Verification items for the finished model (mm, model axes). A direction names the side the tool comes from. Give positions to 0.01 mm unless a question says otherwise; leave off trailing zeros. Order: outer loops, then holes, each group sorted by start corner. A loop starts at its lowest first (then second) coordinate and runs counter-clockwise, first axis right, second up. Notation, with made-up numbers: (22, 83.25) -> (66, 83.25) arc R21 ccw to (66, 88.25) -> close; hole circle Ø4 at (70, -40). An arc over 180 degrees is marked (long way). One line per question, with ' | ' between items. Start each with the question number.
Q1. Section check C-C on z = 12.5. Record the cut outline in (x, y).
Q2. Mould release check, pull along Y, two halves, no side actions. Record for faces 1 (the flat face through (4.623, 7.515, 7.395)), 2 (the flat face through (-8.3, -3, 7)), 3 (the cylindrical face through (-6.77, 10.01, 7.4)): released by +Y, released by -Y, zero draft, split by the parting line, or undercut.
Q3. Access from +Z, -Z, +X, -X, +Y, -Y to the whole of each face (thin tool, end or side, straight path). Record for faces 4 (the flat face through (-1.3, -7, 7)), 5 (the flat face through (-2, -3.1, 7)), 6 (the flat face through (12.263, 9.56, 7.395)).
Q4. Section check D-D on x = -4. Record the cut outline in (y, z).
Q5. Section check B-B on y = 8.5. Record the cut outline in (x, z).
Q6. Section check A-A on y = -4.75. Record the cut outline in (x, z), plus the area to 3 significant figures.
Q7. Material ranges on probe 1 along X at (y, z) = (1, 2.25); probe 2 along X at (y, z) = (-7.5, 8.75); probe 3 along Y at (x, z) = (-6.5, 6.75), recorded low to high. Write a range as [from, to].
Q8. Go/stop test with flat-tipped pins: pin 1 (1.6 mm diameter, centred on x = -2.5, z = 6, fed in from +Y); pin 2 (1.2 mm diameter, centred on y = 2, z = 10.5, fed in from +X); pin 3 (7.5 mm diameter, centred on y = -7.5, z = 8, fed in from +X). Record where each tip stops, or that it passes through.
from build123d import *

# Parameters (mm, degrees)
F0_W     = 2
F0_H     = 4
F1_DEPTH = 15
F2_W     = 2
F2_H     = 4
F3_DEPTH = 15


# Not quite as in the source:
# - a feature names something its author has since deleted; it is built from what else it names


with BuildPart() as f1:
    # F0 (on Top) → F1 (new body)
    with BuildSketch(Plane.XY):
        with BuildLine():
            Line((7, 32.0000030547), (2, 32.0000030547))
            Line((2, 32.0000030547), (2, 43.0000030547))
            ThreePointArc((2, 43.0000030547), (4.22965477, 48.1459058579), (9.7375987459, 49.20147642))
            Line((9.7375987459, 49.20147642), (10.3227891625, 51.113949211))
            ThreePointArc((10.3227891625, 51.113949211), (3.4424209582, 50.0513163902), (0, 44.0000030547))
            Line((0, 44.0000030547), (0, 30.0000030547))
            Line((0, 30.0000030547), (9, 30.0000030547))
            Line((9, 30.0000030547), (9, 37.0000030547))
            Line((9, 37.0000030547), (7, 37.0000030547))
            Line((7, 37.0000030547), (7, 32.0000030547))
        make_face()
        Polygon((10.3227891625, 51.113949211), (9.7375987459, 49.20147642), (20.2561990964, 45.9829291287), (20.841389513, 47.8954019197), align=None)
        with BuildLine():
            Line((20.841389513, 47.8954019197), (20.2561990964, 45.9829291287))
            ThreePointArc((20.2561990964, 45.9829291287), (20.7938383415, 45.6028219427), (21, 44.9774941877))
            Line((21, 44.9774941877), (23, 44.9774941877))
            ThreePointArc((23, 44.9774941877), (22.9273260191, 45.6394915882), (22.7127657141, 46.2699564496))
            ThreePointArc((22.7127657141, 46.2699564496), (22.1205825647, 47.1207678466), (21.277739528, 47.7242382529))
            ThreePointArc((21.277739528, 47.7242382529), (21.0628558439, 47.8182107047), (20.841389513, 47.8954019197))
        make_face()
        with Locations((22, 42.9774941877)):
            Rectangle(F0_W, F0_H)
        with BuildLine():
            Line((23.8132360697, 51.5414804224), (21.277739528, 47.7242382529))
            ThreePointArc((21.277739528, 47.7242382529), (22.1205825647, 47.1207678466), (22.7127657141, 46.2699564496))
            Line((22.7127657141, 46.2699564496), (25.4792139424, 50.4349011311))
            Line((25.4792139424, 50.4349011311), (23.8132360697, 51.5414804224))
        make_face()
    extrude(amount=F1_DEPTH)


with BuildPart() as f3:
    # F2 (on Top) → F3 (new body)
    with BuildSketch(Plane.XY):
        with Locations((-37.8, -36.9225088671)):
            Rectangle(F2_W, F2_H)
        with BuildLine():
            ThreePointArc((-39.5438009036, -33.9170739261), (-39.0061616585, -34.2971811121), (-38.8, -34.9225088671))
            Line((-38.8, -34.9225088671), (-36.8, -34.9225088671))
            ThreePointArc((-36.8, -34.9225088671), (-36.8726739809, -34.2605114665), (-37.0872342859, -33.6300466052))
            ThreePointArc((-37.0872342859, -33.6300466052), (-37.6794174353, -32.7792352081), (-38.522260472, -32.1757648018))
            ThreePointArc((-38.522260472, -32.1757648018), (-38.7371441561, -32.0817923501), (-38.958610487, -32.0046011351))
            Line((-38.958610487, -32.0046011351), (-39.5438009036, -33.9170739261))
        make_face()
        Polygon((-50.0624012541, -30.6985266348), (-39.5438009036, -33.9170739261), (-38.958610487, -32.0046011351), (-49.4772108375, -28.7860538438), align=None)
        with BuildLine():
            ThreePointArc((-57.8, -36.9), (-55.57034523, -31.7540971969), (-50.0624012541, -30.6985266348))
            Line((-50.0624012541, -30.6985266348), (-49.4772108375, -28.7860538438))
            ThreePointArc((-49.4772108375, -28.7860538438), (-56.3575790418, -29.8486866645), (-59.8, -35.9))
            Line((-59.8, -35.9), (-59.8, -49.9))
            Line((-59.8, -49.9), (-50.8, -49.9))
            Line((-50.8, -49.9), (-50.8, -42.9))
            Line((-50.8, -42.9), (-52.8, -42.9))
            Line((-52.8, -42.9), (-52.8, -47.9))
            Line((-52.8, -47.9), (-57.8, -47.9))
            Line((-57.8, -47.9), (-57.8, -36.9))
        make_face()
        with BuildLine():
            ThreePointArc((-38.522260472, -32.1757648018), (-37.6794174353, -32.7792352081), (-37.0872342859, -33.6300466052))
            Line((-37.0872342859, -33.6300466052), (-34.3207860576, -29.4651019236))
            Line((-34.3207860576, -29.4651019236), (-35.9867639303, -28.3585226323))
            Line((-35.9867639303, -28.3585226323), (-38.522260472, -32.1757648018))
        make_face()
    extrude(amount=F3_DEPTH)


with BuildPart() as f3b:
    # F2 (on Top) → F3, piece 2 (new body)
    with BuildSketch(Plane.XY):
        with Locations((33.034186706, 0.0025241677)):
            Rectangle(F2_W, F2_H)
        with BuildLine():
            ThreePointArc((31.2903858024, 3.0079591087), (31.8280250475, 2.6278519227), (32.034186706, 2.0025241677))
            Line((32.034186706, 2.0025241677), (34.034186706, 2.0025241677))
            ThreePointArc((34.034186706, 2.0025241677), (33.9615127251, 2.6645215683), (33.7469524201, 3.2949864296))
            ThreePointArc((33.7469524201, 3.2949864296), (33.1547692707, 4.1457978267), (32.311926234, 4.749268233))
            ThreePointArc((32.311926234, 4.749268233), (32.0970425499, 4.8432406847), (31.875576219, 4.9204318997))
            Line((31.875576219, 4.9204318997), (31.2903858024, 3.0079591087))
        make_face()
        Polygon((20.7717854519, 6.2265064), (31.2903858024, 3.0079591087), (31.875576219, 4.9204318997), (21.3569758685, 8.138979191), align=None)
        with BuildLine():
            ThreePointArc((13.034186706, 0.0250330348), (15.2638414761, 5.1709358379), (20.7717854519, 6.2265064))
            Line((20.7717854519, 6.2265064), (21.3569758685, 8.138979191))
            ThreePointArc((21.3569758685, 8.138979191), (14.4766076642, 7.0763463703), (11.034186706, 1.0250330348))
            Line((11.034186706, 1.0250330348), (11.034186706, -12.9749669652))
            Line((11.034186706, -12.9749669652), (20.034186706, -12.9749669652))
            Line((20.034186706, -12.9749669652), (20.034186706, -5.9749669652))
            Line((20.034186706, -5.9749669652), (18.034186706, -5.9749669652))
            Line((18.034186706, -5.9749669652), (18.034186706, -10.9749669652))
            Line((18.034186706, -10.9749669652), (13.034186706, -10.9749669652))
            Line((13.034186706, -10.9749669652), (13.034186706, 0.0250330348))
        make_face()
        with BuildLine():
            ThreePointArc((32.311926234, 4.749268233), (33.1547692707, 4.1457978267), (33.7469524201, 3.2949864296))
            Line((33.7469524201, 3.2949864296), (36.5134006484, 7.4599311112))
            Line((36.5134006484, 7.4599311112), (34.8474227758, 8.5665104025))
            Line((34.8474227758, 8.5665104025), (32.311926234, 4.749268233))
        make_face()
    extrude(amount=F3_DEPTH)


with BuildPart() as f3c:
    # F2 (on Top) → F3, piece 3 (new body)
    with BuildSketch(Plane.XY):
        with Locations((-12.8, -36.9225088671)):
            Rectangle(F2_W, F2_H)
        with BuildLine():
            ThreePointArc((-14.5438009036, -33.9170739261), (-14.0061616585, -34.2971811121), (-13.8, -34.9225088671))
            Line((-13.8, -34.9225088671), (-11.8, -34.9225088671))
            ThreePointArc((-11.8, -34.9225088671), (-11.8726739809, -34.2605114665), (-12.0872342859, -33.6300466052))
            ThreePointArc((-12.0872342859, -33.6300466052), (-12.6794174353, -32.7792352081), (-13.522260472, -32.1757648018))
            ThreePointArc((-13.522260472, -32.1757648018), (-13.7371441561, -32.0817923501), (-13.958610487, -32.0046011351))
            Line((-13.958610487, -32.0046011351), (-14.5438009036, -33.9170739261))
        make_face()
        Polygon((-25.0624012541, -30.6985266348), (-14.5438009036, -33.9170739261), (-13.958610487, -32.0046011351), (-24.4772108375, -28.7860538438), align=None)
        with BuildLine():
            ThreePointArc((-32.8, -36.9), (-30.57034523, -31.7540971969), (-25.0624012541, -30.6985266348))
            Line((-25.0624012541, -30.6985266348), (-24.4772108375, -28.7860538438))
            ThreePointArc((-24.4772108375, -28.7860538438), (-31.3575790418, -29.8486866645), (-34.8, -35.9))
            Line((-34.8, -35.9), (-34.8, -49.9))
            Line((-34.8, -49.9), (-25.8, -49.9))
            Line((-25.8, -49.9), (-25.8, -42.9))
            Line((-25.8, -42.9), (-27.8, -42.9))
            Line((-27.8, -42.9), (-27.8, -47.9))
            Line((-27.8, -47.9), (-32.8, -47.9))
            Line((-32.8, -47.9), (-32.8, -36.9))
        make_face()
        with BuildLine():
            ThreePointArc((-13.522260472, -32.1757648018), (-12.6794174353, -32.7792352081), (-12.0872342859, -33.6300466052))
            Line((-12.0872342859, -33.6300466052), (-9.3207860576, -29.4651019236))
            Line((-9.3207860576, -29.4651019236), (-10.9867639303, -28.3585226323))
            Line((-10.9867639303, -28.3585226323), (-13.522260472, -32.1757648018))
        make_face()
    extrude(amount=F3_DEPTH)


with BuildPart() as f3d:
    # F2 (on Top) → F3, piece 4 (new body)
    with BuildSketch(Plane.XY):
        with Locations((58.034186706, 0.0025241677)):
            Rectangle(F2_W, F2_H)
        with BuildLine():
            ThreePointArc((56.2903858024, 3.0079591087), (56.8280250475, 2.6278519227), (57.034186706, 2.0025241677))
            Line((57.034186706, 2.0025241677), (59.034186706, 2.0025241677))
            ThreePointArc((59.034186706, 2.0025241677), (58.9615127251, 2.6645215683), (58.7469524201, 3.2949864296))
            ThreePointArc((58.7469524201, 3.2949864296), (58.1547692707, 4.1457978267), (57.311926234, 4.749268233))
            ThreePointArc((57.311926234, 4.749268233), (57.0970425499, 4.8432406847), (56.875576219, 4.9204318997))
            Line((56.875576219, 4.9204318997), (56.2903858024, 3.0079591087))
        make_face()
        Polygon((45.7717854519, 6.2265064), (56.2903858024, 3.0079591087), (56.875576219, 4.9204318997), (46.3569758685, 8.138979191), align=None)
        with BuildLine():
            ThreePointArc((38.034186706, 0.0250330348), (40.2638414761, 5.1709358379), (45.7717854519, 6.2265064))
            Line((45.7717854519, 6.2265064), (46.3569758685, 8.138979191))
            ThreePointArc((46.3569758685, 8.138979191), (39.4766076642, 7.0763463703), (36.034186706, 1.0250330348))
            Line((36.034186706, 1.0250330348), (36.034186706, -12.9749669652))
            Line((36.034186706, -12.9749669652), (45.034186706, -12.9749669652))
            Line((45.034186706, -12.9749669652), (45.034186706, -5.9749669652))
            Line((45.034186706, -5.9749669652), (43.034186706, -5.9749669652))
            Line((43.034186706, -5.9749669652), (43.034186706, -10.9749669652))
            Line((43.034186706, -10.9749669652), (38.034186706, -10.9749669652))
            Line((38.034186706, -10.9749669652), (38.034186706, 0.0250330348))
        make_face()
        with BuildLine():
            ThreePointArc((57.311926234, 4.749268233), (58.1547692707, 4.1457978267), (58.7469524201, 3.2949864296))
            Line((58.7469524201, 3.2949864296), (61.5134006484, 7.4599311112))
            Line((61.5134006484, 7.4599311112), (59.8474227758, 8.5665104025))
            Line((59.8474227758, 8.5665104025), (57.311926234, 4.749268233))
        make_face()
    extrude(amount=F3_DEPTH)


with BuildPart() as f3e:
    # F2 (on Top) → F3, piece 5 (new body)
    with BuildSketch(Plane.XY):
        with Locations((12.2, -36.9225088671)):
            Rectangle(F2_W, F2_H)
        with BuildLine():
            ThreePointArc((10.4561990964, -33.9170739261), (10.9938383415, -34.2971811121), (11.2, -34.9225088671))
            Line((11.2, -34.9225088671), (13.2, -34.9225088671))
            ThreePointArc((13.2, -34.9225088671), (13.1273260191, -34.2605114665), (12.9127657141, -33.6300466052))
            ThreePointArc((12.9127657141, -33.6300466052), (12.3205825647, -32.7792352081), (11.477739528, -32.1757648018))
            ThreePointArc((11.477739528, -32.1757648018), (11.2628558439, -32.0817923501), (11.041389513, -32.0046011351))
            Line((11.041389513, -32.0046011351), (10.4561990964, -33.9170739261))
        make_face()
        Polygon((-0.0624012541, -30.6985266348), (10.4561990964, -33.9170739261), (11.041389513, -32.0046011351), (0.5227891625, -28.7860538438), align=None)
        with BuildLine():
            ThreePointArc((-7.8, -36.9), (-5.57034523, -31.7540971969), (-0.0624012541, -30.6985266348))
            Line((-0.0624012541, -30.6985266348), (0.5227891625, -28.7860538438))
            ThreePointArc((0.5227891625, -28.7860538438), (-6.3575790418, -29.8486866645), (-9.8, -35.9))
            Line((-9.8, -35.9), (-9.8, -49.9))
            Line((-9.8, -49.9), (-0.8, -49.9))
            Line((-0.8, -49.9), (-0.8, -42.9))
            Line((-0.8, -42.9), (-2.8, -42.9))
            Line((-2.8, -42.9), (-2.8, -47.9))
            Line((-2.8, -47.9), (-7.8, -47.9))
            Line((-7.8, -47.9), (-7.8, -36.9))
        make_face()
        with BuildLine():
            ThreePointArc((11.477739528, -32.1757648018), (12.3205825647, -32.7792352081), (12.9127657141, -33.6300466052))
            Line((12.9127657141, -33.6300466052), (15.6792139424, -29.4651019236))
            Line((15.6792139424, -29.4651019236), (14.0132360697, -28.3585226323))
            Line((14.0132360697, -28.3585226323), (11.477739528, -32.1757648018))
        make_face()
    extrude(amount=F3_DEPTH)


with BuildPart() as f1_1:
    # F5: moved
    add(f1.part.moved(Location((-10.3, -40.1, 0))))


solid = f1_1.part
Filled in:
1) outline: (-10.3, -10.1) -> (-1.3, -10.1) -> (-1.3, -3.1) -> (-3.3, -3.1) -> (-3.3, -8.1) -> (-8.3, -8.1) -> (-8.3, 2.9) arc R6 cw to (-0.56, 9.1) -> (9.96, 5.88) arc R1.05 cw to (10.7, 4.88) -> (10.7, 0.88) -> (12.7, 0.88) -> (12.7, 4.88) arc R3.05 ccw to (12.41, 6.17) -> (15.18, 10.33) -> (13.51, 11.44) -> (10.98, 7.62) arc R3.05 ccw to (10.54, 7.8) -> (0.02, 11.01) arc R8 ccw to (-10.3, 3.9) -> close
2) face 1: released by -Y | face 2: undercut | face 3: released by +Y
3) face 4: +Z, -Z, +X, -Y | face 5: +Z, -Z, +X | face 6: +Z, -Z, +Y
4) outline: (-10.1, 0) -> (-8.1, 0) -> (-8.1, 15) -> (-10.1, 15) -> close; (9.12, 0) -> (11.19, 0) -> (11.19, 15) -> (9.12, 15) -> close
5) outline: (-8.45, 0) -> (-5.42, 0) -> (-5.42, 15) -> (-8.45, 15) -> close; (1.4, 0) -> (8.24, 0) -> (8.24, 15) -> (1.4, 15) -> close; (11.56, 0) -> (13.96, 0) -> (13.96, 15) -> (11.56, 15) -> close
6) outline: (-10.3, 0) -> (-8.3, 0) -> (-8.3, 15) -> (-10.3, 15) -> close; (-3.3, 0) -> (-1.3, 0) -> (-1.3, 15) -> (-3.3, 15) -> close | area: 60.0 mm²
7) probe 1: [-10.3, -8.3], [10.7, 12.7] | probe 2: [-10.3, -8.3], [-3.3, -1.3] | probe 3: [-10.1, -8.1], [7.67, 10.18]
8) pin 1: y = 11.36 | pin 2: x = 12.7 | pin 3: x = -1.3
